For this review, take the finished solid that the model builds, in its own axes (mm). Round coordinates to 2 decimals unless told otherwise and drop trailing zeros. Loops run counter-clockwise (first coordinate to the right, second up) from the corner with the lowest first, then second, coordinate; pieces in that order, holes last.
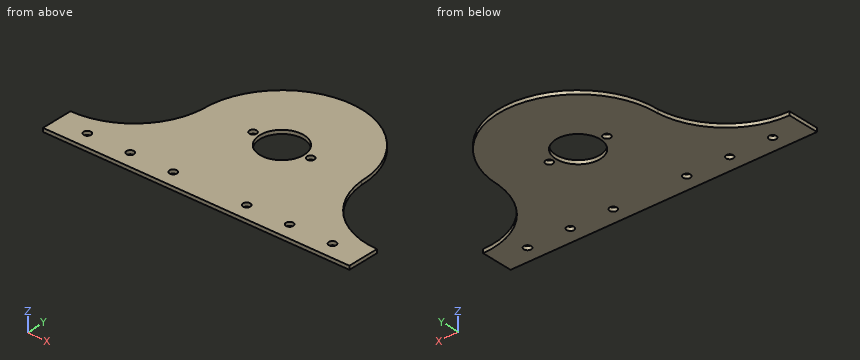
```python
from build123d import *

# Parameters (mm, degrees)
F0_R     = 3
F0_R_2   = 18
F1_DEPTH = 3


with BuildPart() as f1:
    # F0 (on Top) → F1 (new body)
    with BuildSketch(Plane.XY):
        with BuildLine():
            ThreePointArc((125, -55), (84.302949, -39.169511), (65, 0))
            ThreePointArc((65, 0), (0, 65), (-65, 0))
            ThreePointArc((-65, 0), (-84.302949, -39.169511), (-125, -55))
            Line((-125, -55), (-125, -81))
            Line((-125, -81), (125, -81))
            Line((125, -81), (125, -55))
        make_face()
        with Locations((-100, -68)):
            Circle(F0_R, mode=Mode.SUBTRACT)
        with Locations((-65, -68)):
            Circle(F0_R, mode=Mode.SUBTRACT)
        with Locations((-30, -68)):
            Circle(F0_R, mode=Mode.SUBTRACT)
        with Locations((30, -68)):
            Circle(F0_R, mode=Mode.SUBTRACT)
        with Locations((65, -68)):
            Circle(F0_R, mode=Mode.SUBTRACT)
        with Locations((100, -68)):
            Circle(F0_R, mode=Mode.SUBTRACT)
        with Locations((-23.5, 0)):
            Circle(F0_R, mode=Mode.SUBTRACT)
        Circle(F0_R_2, mode=Mode.SUBTRACT)
        with Locations((23.5, 0)):
            Circle(F0_R, mode=Mode.SUBTRACT)
    extrude(amount=F1_DEPTH)


solid = f1.part
```
(1) For L1, parallel to Y at x = 102, z = 0.9; L2, parallel to Y at x = -30, z = 0.95; L3, parallel to X at y = -9, z = 1.2, list the stretches that pass through material, from the lowest coordinate up.
(2) Add section B-B (z = 1.75). Give the number of separate pieces and of enclosed holes in the cut face, plus the area to 3 significant figures.
(3) Add section D-D (y = 27.5). Give the boundary of the cut face in (x, z).
(4) Add section A-A (x = 0). Give the boundary of the cut face in (y, z), plus the area to 3 significant figures.
(5) Add section C-C (x = 30). Give the boundary of the cut face in (y, z), plus the area to 3 significant figures.
(6) Insertion check: pin 1 Ø1.5 at (y, z) = (24, 1) entering from +X. The pin has a flat end and moves straight along its axis. Give the tip position at first contact, or say it passes through.
Outcome:
1. L1: y = -81 to -70.24, -65.76 to -50.44
1. L2: y = -81 to -71, -65 to 57.66
1. L3: x = -66.48 to -15.59, 15.59 to 66.48
2. separate pieces: 1
2. enclosed holes: 9
2. area: 20,600 mm2
3. outline: (-58.9, 0) - (58.9, 0) - (58.9, 3) - (-58.9, 3) - close
4. outline: (-81, 0) - (-18, 0) - (-18, 3) - (-81, 3) - close; (18, 0) - (65, 0) - (65, 3) - (18, 3) - close
4. area: 330 mm2
5. outline: (-81, 0) - (-71, 0) - (-71, 3) - (-81, 3) - close; (-65, 0) - (57.66, 0) - (57.66, 3) - (-65, 3) - close
5. area: 398 mm2
6. pin 1: stops at x = 60.7
